from build123d import *

# Parameters (mm, degrees)
SKETCH1_R               = 7.6
SKETCH1_R_2             = 3
SKETCH1_W               = 10
SKETCH1_H               = 3.15
BOSS_EXTRUDE1_DEPTH     = 3
FILLET1_R               = 10
SKETCH2_W               = 3.2
SKETCH2_H               = 6
SKETCH2_H_2             = 2.5
SKETCH2_W_2             = 1
SKETCH2_H_3             = 2
CUT_EXTRUDE1_DEPTH      = 1
CUT_EXTRUDE1_DEPTH_BACK = 4


with BuildPart() as part:
    # Sketch1 → Boss-Extrude1 (new body)
    with BuildSketch(Plane(origin=(0, 0, 0), x_dir=(0, 0, -1), z_dir=(1, 0, 0))):
        Polygon((102.223805307, 6), (123.223805307, 6), (102.223805307, 27), align=None)
        Polygon((102.223805307, 6), (123.223805307, 6), (123.223805307, -9), (107.223805307, -9), (107.223805307, 0), (30, 0), (30, -9), (12.5, -9), (12.5, 0), (0, 0), (0, 46), (20.444761061, 46), (20.444761061, 43), (40.889522123, 43), (40.889522123, 46), (61.334283184, 46), (61.334283184, 43), (81.779044246, 43), (81.779044246, 46), (102.223805307, 46), align=None)
        with Locations((84.723805307, 21)):
            Circle(SKETCH1_R, mode=Mode.SUBTRACT)
        with Locations((51.111902654, 17.95)):
            Circle(SKETCH1_R, mode=Mode.SUBTRACT)
        with Locations((17.5, 14.9)):
            Circle(SKETCH1_R_2, mode=Mode.SUBTRACT)
        with Locations((115.223805307, -4.575)):
            Rectangle(SKETCH1_W, SKETCH1_H, mode=Mode.SUBTRACT)
        with Locations((21.25, -4.575)):
            Rectangle(SKETCH1_W, SKETCH1_H, mode=Mode.SUBTRACT)
    extrude(amount=BOSS_EXTRUDE1_DEPTH)

    # Fillet1
    fillet1_edges = [part.edges().sort_by_distance(p)[0] for p in [
        (1.5, 6, -123.223805307),
        (1.5, 27, -102.223805307),
    ]]
    fillet(fillet1_edges, radius=FILLET1_R)

    # Sketch2 → Cut-Extrude1 (cut, two sides)
    with BuildSketch(Plane(origin=(3, 0, 0), x_dir=(0, 0, -1), z_dir=(1, 0, 0))) as cut_extrude1_sk:
        with Locations((51.111902654, 38.5)):
            Rectangle(SKETCH2_W, SKETCH2_H)
        with Locations((51.111902654, 42.75)):
            Rectangle(SKETCH2_W, SKETCH2_H_2)
        with Locations((49.011902654, 42.75)):
            Rectangle(SKETCH2_W_2, SKETCH2_H_2)
        with Locations((51.111902654, 45)):
            Rectangle(SKETCH2_W, SKETCH2_H_3)
        with Locations((53.211902654, 42.75)):
            Rectangle(SKETCH2_W_2, SKETCH2_H_2)
    extrude(amount=CUT_EXTRUDE1_DEPTH, mode=Mode.SUBTRACT)
    extrude(cut_extrude1_sk.sketch, amount=-CUT_EXTRUDE1_DEPTH_BACK, mode=Mode.SUBTRACT)


solid = part.part
Part model, mm, in its own coordinate system. A direction names the side the tool comes from. Give positions to 0.01 mm unless a question says otherwise; leave off trailing zeros. Loops run counter-clockwise (first coordinate to the right, second up) from the corner with the lowest first, then second, coordinate; pieces in that order, holes last.
(1) 3-axis set-ups, long thin cutter, end or side, ignore diameter. For faces 1 (the flat face through (1, 39, -102.224)), 2 (the flat face through (1, -5, -16.25)), 3 (the flat face through (2, 38, -52.712)), 4 (the flat face through (1, 46, -57)), 5 (the flat face through (1, -5, -107.224)): which of +Z, -Z, +X, -X, +Y, -Y reach the whole face in a straight line?
Return value:
face 1: -Z, +X, -X, +Y
face 2: +X, -X
face 3: +X, -X, +Y
face 4: +Z, -Z, +X, -X, +Y
face 5: +X, -X, -Y
(2) Band-saw the part on B-B (y = 21). Write the cut outline in (x, z), and give its area (3 significant figures).
Return value:
outline: (0, -108.22) - (3, -108.22) - (3, -92.32) - (0, -92.32) - close; (0, -77.12) - (3, -77.12) - (3, -58.07) - (0, -58.07) - close; (0, -44.15) - (3, -44.15) - (3, 0) - (0, 0) - close
area: 237 mm2
(3) Drill centre lines: line 1 along Y through (x, z) = (1, -17.5); line 2 along Z through (x, y) = (0.45, -6); line 3 along Y through (x, z) = (2.8, -24.5). Where is each one in solid material? Low to high.
Return value:
line 1: y = -9 to -6.15, -3 to 11.9, 17.9 to 46
line 2: z = -123.22 to -120.22, -110.22 to -107.22, -30 to -26.25, -16.25 to -12.5
line 3: y = -9 to -6.15, -3 to 43
(4) Pull direction Y, two halves, no side cores. Call faces 6 (the flat face through (1, -5, -26.25)), 7 (the flat face through (1.479, 16.394, -112.83)), 8 (the flat face through (3, 19, -61)): pulls with the +Y half, pulls with the -Y half, needs draft (parallel to the pull), parting line crosses it, or undercut.
Return value:
face 6: undercut
face 7: pulls with the +Y half
face 8: needs draft
(5) Band-saw the part on D-D (z = -31.5). Write the cut outline in (x, y), and give its area (3 significant figures).
Return value:
outline: (0, 0) - (3, 0) - (3, 43) - (0, 43) - close
area: 129 mm2
(6) Band-saw the part on C-C (x = 1.1). Count the separate pieces of the cut face and the enclosed holes in it, and give its area (3 significant figures).
Return value:
separate pieces: 1
enclosed holes: 5
area: 4,730 mm2
(7) Pin check, flat tips, straight feed: pin 1 (0.5 mm diameter, centred on x = 2, z = -49, fed in from -Y); pin 2 (0.9 mm diameter, centred on x = 2, y = 44.5, fed in from -Z); pin 3 (12 mm diameter, centred on y = 21, z = -84.72, fed in from -X). Stop position of each tip, or through.
Return value:
pin 1: stops at y = 0
pin 2: stops at z = -102.22
pin 3: passes through
(8) Band-saw the part on A-A (y = 14.9). Write the cut outline in (x, z), and give its area (3 significant figures).
Return value:
outline: (0, -114.32) - (3, -114.32) - (3, -89.26) - (0, -89.26) - close; (0, -80.19) - (3, -80.19) - (3, -58.07) - (0, -58.07) - close; (0, -44.15) - (3, -44.15) - (3, -20.5) - (0, -20.5) - close; (0, -14.5) - (3, -14.5) - (3, 0) - (0, 0) - close
area: 256 mm2
